Build history of the part. All positions in model axes, mm. Give positions to 0.01 mm unless a question says otherwise; leave off trailing zeros. One line per item, written item: value.
Autodesk Fusion 360 part; units mm, degrees
sketch "Skizze1" plane through (0, 0, 0) normal (0, 0, 1) x (1, 0, 0)
sketch "Skizze2" plane through (0, 0, 0) normal (0, 0, 1) x (1, 0, 0)
  circle A0 centre (0, 0) radius 5
extrude "Extrusion1" add sketch "Skizze2" against normal blind 5
fillet "Abrundung1" radius 5 1 edges at (-4.6616, 1.8081, -5)
sketch "Skizze3" plane through (0, 0, 0) normal (0, 0, 1) x (-1, 0, 0)
  circle A0 centre (0, 0) radius 5
  circle A1 centre (0, 0) radius 1.525
  dimension "d5" = 3.05
extrude "Extrusion2" add sketch "Skizze3" along normal blind 2
extrude "Extrusion3" cut 1 faces at (0.5137, -0.5901, 0) along direction (0, 0, -1) blind 4
1) Mould opens along X. For faces 1 (the face through (1.524, 0.067, -1.042)), 2 (the face through (1.2, -1.2, 2)) say: released by +X, released by -X, zero draft, split by the parting line, or undercut.
Check values:
face 1: undercut
face 2: zero draft
2) Drill centre lines: probe 1 along X at (y, z) = (0, 0.7) (3 decimals); probe 2 along Y at (x, z) = (0, -2.5) (3 decimals). Where is each one in solid material? Low to high. Write a range as from..to.
Check values:
probe 1: -5..-1.525, 1.525..5
probe 2: -4.331..-1.525, 1.525..4.331
3) Pin check, flat tips, straight feed: pin 1 (1.5 mm diameter, centred on x = 2.5, z = 0, fed in from +Y); pin 2 (6 mm diameter, centred on x = -2, y = 4, fed in from -Z). Stop position of each tip, or through.
Check values:
pin 1: y = 4.68
pin 2: z = -4.78
